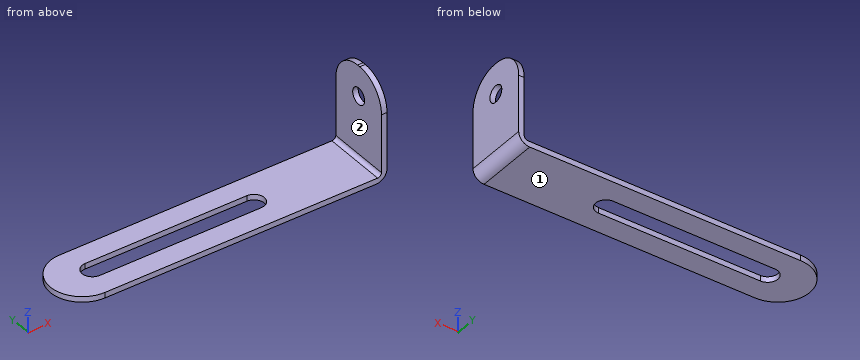
Autodesk Inventor part; units mm, degrees
ref_plane "YZ Plane" through (0, 0, 0) normal (1, 0, 0) x (0, 1, 0)
ref_plane "XZ Plane" through (0, 0, 0) normal (0, 1, 0) x (-1, 0, 0)
ref_plane "XY Plane" through (0, 0, 0) normal (0, 0, 1) x (1, 0, 0)
sketch "Esboço1" plane through (0, 0, 0) normal (0, 0, 1) x (1, 0, 0)
  line L0 (-18.5827, 6.5782) -> (32.5173, 6.5782)
  line L1 (-18.5827, -4.9718) -> (32.5173, -4.9718)
  line L2 (32.5173, -4.9718) -> (32.5173, 6.5782)
  arc A0 (-18.5827, 6.5782) -> (-18.5827, -4.9718) centre (-18.5827, 0.8032) ccw
  line L3 (-16.7327, 2.6532) -> (12.5673, 2.6532)
  line L4 (12.5673, -1.0468) -> (-16.7327, -1.0468)
  arc A1 (-16.7327, 2.6532) -> (-16.7327, -1.0468) centre (-16.7327, 0.8032) ccw
  arc A2 (12.5673, -1.0468) -> (12.5673, 2.6532) centre (12.5673, 0.8032) ccw
  point P0 (0, 0)
  point P1 (-2.0827, 0.8032)
  point P2 (-2.0827, 0.8032)
extrude "Extrusão1" add sketch "Esboço1" along normal blind 1
sketch "Esboço2" plane through (0, 0, 1) normal (0, 0, 1) x (1, 0, 0)
  line L0 (32.5173, 6.5782) -> (31.5173, 6.5782)
  line L1 (31.5173, 6.5782) -> (31.5173, -4.9718)
  line L2 (31.5173, -4.9718) -> (32.5173, -4.9718)
  line L3 (32.5173, -4.9718) -> (32.5173, 6.5782)
  point P0 (0, 0)
  dimension "d8" = 1
extrude "Extrusão2" add sketch "Esboço2" along normal blind 16.7
fillet "Arredondamento1" radius 5.5 1 edges at (32.0173, 6.5782, 17.7)
fillet "Arredondamento2" radius 5.5 1 edges at (32.0173, -4.9718, 17.7)
sketch "Esboço3" plane through (32.5173, -4.9718, 0) normal (1, 0, 0) x (0, 0, -1)
  circle A0 centre (-12.2, 5.775) radius 1.5
  line L0 (0, 11.55) -> (0, 0)
  point P0 (0, 4.9718)
  dimension "d25" = 12.2
hole "Furo1" at (32.5173, 0.8032, 12.2) direction (-1, 0, 0) diameter 3 end through all
fillet "Fillet3" radius 0.7 1 edges at (31.5173, 0.8032, 1)
fillet "Fillet4" radius 2 1 edges at (32.5173, 0.8032, 0)
equation "\"BendRadius\" = Thickness"
equation "\"BendReliefWidth\" = Thickness"
equation "\"BendReliefDepth\" = 0.5 * Thickness"
equation "\"CornerReliefSize\" = 4 * Thickness"
equation "\"MinimumRemnant\" = 2 * Thickness"
equation "\"TransitionRadius\" = BendRadius"
equation "\"JacobiRadiusSize\" = Thickness"
equation "\"GapSize\" = Thickness"
properties part number "apoio de escudo2"
Design review of the part built by this model. Coordinates are the model's own, in mm. Face numbers are marked on the shaded views. A direction names the side the tool comes from. Coordinates: 2 decimals unless noted, no trailing zeros. Order: outer loops, then holes, each group sorted by start corner. A loop starts at its lowest first (then second) coordinate and runs counter-clockwise, first axis right, second up.
1) Take a section at C-C, the plane x = 26.5. Give the boundary of the cut face in (y, z).
2) For the marked faces 1 and 2, list the 3-axis set-ups (+Z, -Z, +X, -X, +Y, -Y) from which the entire face can be reached by the end or side of a thin tool; tool diameter is ignored.
3) Take a section at A-A, the plane x = -10.5. Give the boundary of the cut face in (y, z), and give its area (3 significant figures).
4) Take a section at B-B, the plane y = -3. Give the boundary of the cut face in (x, z), and give its area (3 significant figures).
5) Wall thickness on line 1 along Y through (x, z) = (31.8, 12.2); line 2 along Z through (x, y) = (-7.5, 3.5); line 3 along X through (y, z) = (-2.75, 14.25): over which ranges is each line inside the solid? List them lowest first.
6) Take a section at D-D, the plane z = 8. Give the boundary of the cut face in (x, y), and give its area (4 significant figures).
7) Clearance check with flat-ended pins moving along their axes: pin 1 (3 mm diameter, centred on y = 3.5, z = 7.5, fed in from -X); pin 2 (4 mm diameter, centred on x = 20.5, y = -2.5, fed in from -Z). State where each tip first meets the part, or that it passes through.
Returned:
1. outline: (-4.97, 0) - (6.58, 0) - (6.58, 1) - (-4.97, 1) - close
2. face 1: -Z, +X, -X, +Y, -Y
2. face 2: +Z, -X, +Y, -Y
3. outline: (-4.97, 0) - (-1.05, 0) - (-1.05, 1) - (-4.97, 1) - close; (2.65, 0) - (6.58, 0) - (6.58, 1) - (2.65, 1) - close
3. area: 7.85 mm2
4. outline: (-22.93, 0) - (30.52, 0) arc R2 ccw to (32.52, 2) - (32.52, 16.42) - (31.52, 16.42) - (31.52, 1.7) arc R0.7 cw to (30.82, 1) - (-22.93, 1) - close
4. area: 70.1 mm2
5. line 1: y = -4.97 to -0.7, 2.3 to 6.58
5. line 2: z = 0 to 1
5. line 3: x = 31.52 to 32.52
6. outline: (31.52, -4.97) - (32.52, -4.97) - (32.52, 6.58) - (31.52, 6.58) - close
6. area: 11.55 mm2
7. pin 1: stops at x = 31.52
7. pin 2: stops at z = 0
